Autodesk Inventor part; units mm, degrees
ref_plane "YZ Plane" through (0, 0, 0) normal (1, 0, 0) x (0, 1, 0)
ref_plane "XZ Plane" through (0, 0, 0) normal (0, 1, 0) x (-1, 0, 0)
ref_plane "XY Plane" through (0, 0, 0) normal (0, 0, 1) x (1, 0, 0)
sketch "Sketch1" plane through (0, 0, 0) normal (0, 0, 1) x (1, 0, 0)
  line L0 (-1.39, -1.09) -> (1.39, -1.09)
  line L1 (1.39, -1.09) -> (1.39, -2.09)
  line L2 (1.39, -2.09) -> (-1.39, -2.09)
  line L3 (-1.39, -2.09) -> (-1.39, -1.09)
  point P0 (0, 0)
  dimension "d0" = 1
  dimension "d1" = 1.39
  dimension "d2" = 2.78
  dimension "d3" = 1.09
extrude "Extrusion1" add sketch "Sketch1" along normal blind 15.9
sketch "Sketch2" plane through (-1.39, -1.09, 0) normal (0, 1, 0) x (1, 0, 0)
  line L0 (0, 0) -> (0, -15.9)
  line L1 (0, -8.8) -> (2.78, -8.8)
  line L2 (2.78, -8.8) -> (2.78, -15.9)
  line L3 (2.78, -15.9) -> (0, -15.9)
  line L4 (0, -15.9) -> (0, -8.8)
  point P0 (1.39, 0)
  dimension "d6" = 7.1
extrude "Extrusion2" cut sketch "Sketch2" against normal blind 0.2685
sketch "Sketch3" plane through (0, 0, 0) normal (0, 0, -1) x (-1, 0, 0)
  line L0 (-1.39, -1.09) -> (1.39, -1.09)
  line L1 (1.39, -1.09) -> (1.39, 1.69)
  line L2 (1.39, 1.69) -> (-1.39, 1.69)
  line L3 (-1.39, 1.69) -> (-1.39, -1.09)
  point P0 (0, 0)
  dimension "d9" = 2.78
extrude "Extrusion3" add sketch "Sketch3" against normal blind 2
sketch "Sketch4" plane through (0, 0, 0) normal (0, 0, -1) x (-1, 0, 0)
  line L0 (-1.39, 1.69) -> (-1.39, -2.09)
  line L1 (1.39, -2.09) -> (1.39, 1.69)
  line L2 (1.39, 1.69) -> (-1.39, 1.69)
  circle A0 centre (0, 0) radius 0.8
  line L3 (-1.39, -1.3585) -> (1.39, -1.3585)
  line L4 (-1.39, -1.09) -> (1.39, -1.09)
  line L5 (-1.39, -1.09) -> (-0.7252, 0.3377)
  line L6 (1.39, -1.09) -> (0.7252, 0.3377)
  dimension "d12" = 1.6
extrude "Extrusion4" cut sketch "Sketch4" against normal through all contours L2 L1 L6 A0 L5 L0
sketch "Sketch5" plane through (0, 0, 0) normal (0, 0, -1) x (-1, 0, 0)
  line L0 (-0.7252, 0.3377) -> (-1.39, -1.09)
  line L1 (-1.39, -1.09) -> (-1.39, -2.09)
  line L2 (-1.39, -2.09) -> (1.39, -2.09)
  line L3 (1.39, -2.09) -> (1.39, -1.09)
  line L4 (1.39, -1.09) -> (0.7252, 0.3377)
  arc A0 (0.7252, 0.3377) -> (-0.7252, 0.3377) centre (0, 0) ccw
  circle A1 centre (0, 0) radius 0.8
extrude "Extrusion5" cut sketch "Sketch5" against normal blind 1 contours A1 L4 L3 L2 L1 L0
hole "Hole1" at (0, 0, 0) direction (0, 0, 1) diameter 0.5 depth 1.7 countersink diameter 1 countersink angle 90
sketch "Sketch6" plane through (-1.39, -2.09, 15.9) normal (0, -1, 0) x (1, 0, 0)
  line L0 (2.78, -15.9) -> (2.78, 0)
  line L1 (2.78, 0) -> (0, 0)
  circle A0 centre (1.39, -1.5) radius 0.5
  point P0 (2.78, -14.9)
  point P1 (1.39, -15.9)
  point P2 (1.39, -1)
  point P3 (1.39, -2)
  dimension "d26" = 1
  dimension "d27" = 1.39
  dimension "d28" = 1.5
extrude "Extrusion6" [suppressed]
chamfer "Chamfer1" distance 1 angle 45 1 edges at (0, -2.09, 1)
ref_plane "Work Plane1" through (0, -2.09, 14.9) normal (0, 0, 1) x (1, 0, 0)
ref_plane "Work Plane2" through (0, -2.09, 13.9) normal (0, 0, 1) x (1, 0, 0)
sketch "Sketch10" plane through (0, 0, 15.9) normal (0, 0, 1) x (1, 0, 0)
  line L0 (1.39, -1.3585) -> (-1.39, -1.3585)
  circle A0 centre (0, 0) radius 2.09
  line L1 (1.39, -2.09) -> (-1.39, -2.09)
  dimension "d54" = 4.18
extrude "Extrusion7" add sketch "Sketch10" against normal blind 1
sketch "Sketch11" plane through (0, 0, 15.9) normal (0, 0, 1) x (1, 0, 0)
  arc A0 (1.39, -1.5608) -> (-1.39, -1.5608) centre (0, 0) ccw
  circle A1 centre (0, 0) radius 1.3
  point P0 (1.6431, -0.954)
  point P1 (-1.6431, -0.954)
  dimension "d41" = 2.6
hole "Hole2" at (0, 0, 15.9) direction (0, 0, -1) diameter 3 depth 1.1
fillet "Fillet3" radius 0.7 2 edges at (1.39, -2.09, 8.95) (-1.39, -2.09, 8.95)
sketch "Sketch13" plane through (-1.39, -1.09, 8.8) normal (0, 0, 1) x (1, 0, 0)
  point P0 (1.39, 1.09)
  point P1 (1.39, 1.09)
hole "Hole4" at (0, 0, 8.8) at (0, 0, 8.8) direction (0, 0, -1) diameter 2.8 depth 6.8
sketch "Sketch15" plane through (0, -2.09, 14.9) normal (0, 0, 1) x (1, 0, 0)
  point P0 (0, 2.09)
  point P1 (0, 2.09)
hole "Hole5" [suppressed]
properties part number "MU_Motor_Asm_Frame_new3" material "Aluminum-6061"
Source: CAD feature listing. Evaluate the final solid. Frame: model axes, mm. A direction names the side the tool comes from. Round coordinates to 2 decimals unless told otherwise and drop trailing zeros. Write each loop counter-clockwise with the first axis right and the second up, starting at its lowest first coordinate (ties: lowest second). Pieces come first, ordered by that corner, then holes. Notation, with made-up numbers: M 26.5,-1.75 L 58.5,-1.75 A26 ccw 58.5,35.25 Z; hole C 1.5,38 d11. An arc over 180 degrees is marked long. Use CSV: the item, a comma, the result in double quotes. Start each with the question number.
Q1. Cut plane A-A on x = 0. Output: boundary loops of the cut face in (y, z), plus the area to 3 significant figures.
Q2. Cut plane C-C on z = 6.5. Output: boundary loops of the cut face in (x, y).
Q3. First-contact query: P1, Ø1.1, axis at x = 0.5, y = 0, coming from the +Z side; P2, Ø0.6, axis at x = 1, z = 6.5, coming from the +Y side; P3, Ø2, axis at x = -0.5, z = 13, coming from the +Y side. Flat tips, straight axial feed; report the tip coordinate or a pass-through.
Q4. Access query for faces 1 (the face through (0.104, 0.793, 0.764)), 2 (the face through (1.062, -0.386, 1.493)), 3 (the face through (0, -1.4, 5.4)). Directions: +Z, -Z, +X, -X, +Y, -Y. A direction counts if a zero-diameter tool reaches every point of the face in a straight line with its end or side. Return the directions, or none.
Q5. Cut plane B-B on y = 0. Output: boundary loops of the cut face in (x, z).
Q6. Line query: line 1 (X direction, y = 0, z = 15.6); line 2 (Z direction, x = -1.45, y = 1.1); line 3 (Y direction, x = 0, z = 1.25). Output: solid intervals per line, ascending. Write a range as from..to.
Q7. Pull-direction query (X, two-part tool) for faces 4 (the face through (0, -1.358, 12)), 5 (the face through (0.575, -1.386, 15.342)), 6 (the face through (-1.062, -0.386, 1.493)); classes: +X half, -X half, draft (parallel to the pull), parting line (faces both ways), or undercut.
Results found:
1,outline,"M -2.09,2 L -1.09,1 L -0.8,1 L -0.8,0 L -0.5,0 L -0.25,0.25 L -0.25,1.7 L 0.25,1.7 L 0.25,0.25 L 0.5,0 L 0.8,0 L 0.8,2 L -1.4,2 L -1.4,8.8 L -1.36,8.8 L -1.36,14.8 L -1.5,14.8 L -1.5,15.9 L -2.09,15.9 Z; M 1.5,14.9 L 2.09,14.9 L 2.09,15.9 L 1.5,15.9 Z"
1,area,"13.4 mm^2"
2,outline,"M -1.39,-1.39 A0.7 ccw -0.69,-2.09 L 0.69,-2.09 A0.7 ccw 1.39,-1.39 L 1.39,-1.09 L 0.88,-1.09 A1.4 cw -0.88,-1.09 L -1.39,-1.09 Z"
3,P1,"z = 2"
3,P2,"y = -1.09"
3,P3,"y = -1.36"
4,face 1,"-Z"
4,face 2,"-Z, +X, +Y"
4,face 3,"+Y"
5,outline,"M -2.09,14.9 L -1.5,14.9 L -1.5,15.9 L -2.09,15.9 Z; M -0.88,1 L -0.8,1 L -0.8,0 L -0.5,0 L -0.25,0.25 L -0.25,1.7 L 0.25,1.7 L 0.25,0.25 L 0.5,0 L 0.8,0 L 0.8,1 L 0.88,1 L 0.88,2 L -0.88,2 Z; M 1.5,14.9 L 2.09,14.9 L 2.09,15.9 L 1.5,15.9 Z"
6,line 1,"-2.09..-1.5, 1.5..2.09"
6,line 2,"14.9..15.9"
6,line 3,"-1.34..-0.25, 0.25..0.8"
7,face 4,"draft"
7,face 5,"undercut"
7,face 6,"-X half"
